from build123d import *

# Parameters (mm, degrees)
SKETCH_1_R          = 24
SKETCH_1_R_2        = 22
EXTRUDE_1_DEPTH     = 50
CUT_EXTRUDE_1_DEPTH = 20
CUT_EXTRUDE_2_DEPTH = 74.34848345


with BuildPart() as part:
    # 草图1 → 凸台-拉伸1 (new, symmetric)
    with BuildSketch(Plane.XY):
        Circle(SKETCH_1_R)
        Circle(SKETCH_1_R_2, mode=Mode.SUBTRACT)
    extrude(amount=EXTRUDE_1_DEPTH, both=True)

    # 草图2 → 切除-拉伸1 (cut)
    with BuildSketch(Plane.ZY.offset(24)):
        with BuildLine():
            Line((38, 3), (50, 3))
            Line((50, 3), (50, -3))
            Line((50, -3), (38, -3))
            ThreePointArc((38, -3), (35, 0), (38, 3))
        make_face()
    extrude(amount=-CUT_EXTRUDE_1_DEPTH, mode=Mode.SUBTRACT)

    # 草图3 → 切除-拉伸2 (cut, through all)
    with BuildSketch(Plane(origin=(0, 24, 0), x_dir=(1, 0, 0), z_dir=(0, 1, 0))):
        with BuildLine():
            Line((-4, 13), (-4, 23))
            ThreePointArc((-4, 23), (0, 27), (4, 23))
            Line((4, 23), (4, 13))
            ThreePointArc((4, 13), (0, 9), (-4, 13))
        make_face()
        with BuildLine():
            Line((-4, -39), (-4, -29))
            ThreePointArc((-4, -29), (0, -25), (4, -29))
            Line((4, -29), (4, -39))
            ThreePointArc((4, -39), (0, -43), (-4, -39))
        make_face()
    extrude(amount=-CUT_EXTRUDE_2_DEPTH, mode=Mode.SUBTRACT)


solid = part.part
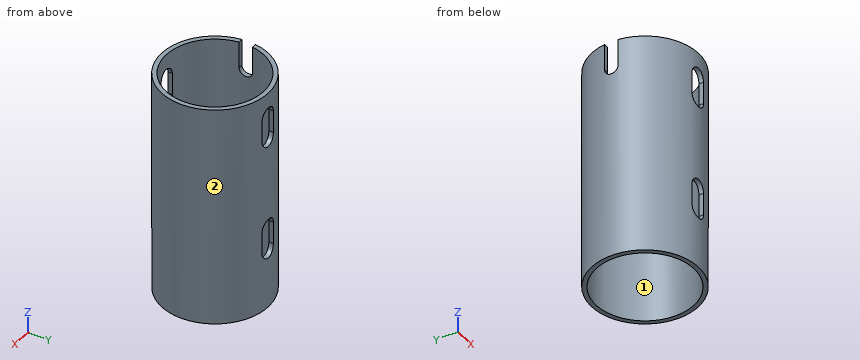
Check sheet for the modelled part. Datum: model origin and axes. Units: mm. Face numbers are marked on the shaded views. Round coordinates to 2 decimals unless told otherwise and drop trailing zeros. Order: outer loops, then holes, each group sorted by start corner. A loop starts at its lowest first (then second) coordinate and runs counter-clockwise, first axis right, second up. Notation, with made-up numbers: M 22.25,-23.75 L 71.25,-23.75 A26 ccw 71.25,-6.75 Z; hole C -39.5,9.5 d7. An arc over 180 degrees is marked long. One line per item, written item: value. Start each with the question number.
1. Scan lines: line 1 along X through (y, z) = (0, 8); line 2 along Y through (x, z) = (-18.5, -16). Record each from-to range of solid material in increasing order.
2. Gauge pin test, flat ends, axial feed: P1, Ø1.6, axis at y = -22.5, z = -20.5, coming from the -X side; P2, Ø0.6, axis at y = -22.5, z = 34, coming from the +X side; P3, Ø1, axis at y = 16, z = 32.5, coming from the -X side. Record the tip position at first contact, or that the pin passes through.
3. Release check for a two-part mould opening along Y. For the marked faces 1 and 2 record: released by +Y, released by -Y, zero draft, split by the parting line, or undercut.
4. Section check B-B on x = 0. Enter the section's corners in (y, z), and give its area (3 significant figures).
5. Section check C-C on x = -13.5. Enter the section's corners in (y, z).
6. Section check D-D on z = -7. Enter the section's corners in (x, y), and give its area (3 significant figures).
7. Section check A-A on y = 4. Enter the section's corners in (x, z), and give its area (3 significant figures).
Results found:
1. line 1: -24 to -22, 22 to 24
1. line 2: -15.29 to -11.91, 11.91 to 15.29
2. P1: x = -10.25
2. P2: x = 9.12
2. P3: x = -18.32
3. face 1: undercut
3. face 2: split by the parting line
4. outline: M -24,-50 L -22,-50 L -22,-27 L -24,-27 Z; M -24,-9 L -22,-9 L -22,25 L -24,25 Z; M -24,43 L -22,43 L -22,50 L -24,50 Z; M 22,-50 L 24,-50 L 24,-27 L 22,-27 Z; M 22,-9 L 24,-9 L 24,25 L 22,25 Z; M 22,43 L 24,43 L 24,50 L 22,50 Z
4. area: 256 mm^2
5. outline: M -19.84,-50 L -17.37,-50 L -17.37,50 L -19.84,50 Z; M 17.37,-50 L 19.84,-50 L 19.84,50 L 17.37,50 Z
6. outline: C 0,0 d48; hole C 0,0 d44
6. area: 289 mm^2
7. outline: M -23.66,-50 L -21.63,-50 L -21.63,50 L -23.66,50 Z; M 21.63,-50 L 23.66,-50 L 23.66,50 L 21.63,50 Z
7. area: 406 mm^2
